Can you work these out from the model? Positions are in its coordinate system, mm. A direction names the side the tool comes from. Coordinates: 2 decimals unless noted, no trailing zeros. Order: outer loops, then holes, each group sorted by start corner. A loop starts at its lowest first (then second) coordinate and runs counter-clockwise, first axis right, second up. Notation, with made-up numbers: M 7.25,73 L 54.25,73 A8 ccw 54.25,87 Z; hole C 83,16 d10. An arc over 180 degrees is marked long. Answer as a JSON object with one key per item and string values.
from build123d import *

# Parameters (mm, degrees)
SKETCH1_R           = 5.0038
BOSS_EXTRUDE1_DEPTH = 12.0904
SKETCH1_5_R         = 6.604
SKETCH1_6_R         = 6.604
BOSS_EXTRUDE2_DEPTH = 3.302
SKETCH2_R           = 2.9972
CUT_EXTRUDE1_DEPTH  = 11.43
SKETCH3_R           = 5.2705
CUT_EXTRUDE2_DEPTH  = 2.9464
SKETCH4_W           = 1.623389838
SKETCH4_H           = 6.759688833
BOSS_EXTRUDE3_DEPTH = 12.192


with BuildPart() as part:
    # Sketch1 → Boss-Extrude1 (new body)
    with BuildSketch(Plane(origin=(0, 0, 0), x_dir=(1, 0, 0), z_dir=(0, 1, 0))):
        with Locations(Location((0, 0, 0), (0, 0, 270))):
            Circle(SKETCH1_R)
    extrude(amount=BOSS_EXTRUDE1_DEPTH)

    # Sketch1_5 → section 0 of loft1
    with BuildSketch(Plane(origin=(0, 0, 0), x_dir=(1, 0, 0), z_dir=(0, 1, 0)), mode=Mode.PRIVATE) as loft1_s0:
        Circle(SKETCH1_5_R)
    # loft up to a face of the part (loft1)
    loft([loft1_s0.sketch, Face(Wire([part.edges().sort_by_distance((3.647613218, 12.0904, -3.425336809))[0]]))])

    # Sketch1_6 → Boss-Extrude2 (add)
    with BuildSketch(Plane(origin=(0, 0, 0), x_dir=(1, 0, 0), z_dir=(0, 1, 0))):
        with Locations(Location((0, 0, 0), (0, 0, 270))):
            Circle(SKETCH1_6_R)
    extrude(amount=-BOSS_EXTRUDE2_DEPTH)

    # Sketch2 → Cut-Extrude1 (cut)
    with BuildSketch(Plane.XZ.offset(3.302)):
        with Locations(Location((0, 0, 0), (0, 0, 270))):
            Circle(SKETCH2_R)
    extrude(amount=-CUT_EXTRUDE1_DEPTH, mode=Mode.SUBTRACT)

    # Sketch3 → Cut-Extrude2 (cut)
    with BuildSketch(Plane.XZ.offset(3.302)):
        with Locations(Location((0, 0, 0), (0, 0, 270))):
            Circle(SKETCH3_R)
    extrude(amount=-CUT_EXTRUDE2_DEPTH, mode=Mode.SUBTRACT)

    # Sketch4 → Boss-Extrude3 (add)
    with BuildSketch(Plane.XZ.offset(0.3556)):
        with Locations((-2.310294919, 0.731856075)):
            Rectangle(SKETCH4_W, SKETCH4_H)
    extrude(amount=-BOSS_EXTRUDE3_DEPTH)


solid = part.part
Item 1: I want a section at B-B, the plane y = 4.25. Write out the boundary of the cut face in (x, z), plus the area to 3 significant figures.
Answers follow:
{"outline": "C 0,0 d12.08; hole M -1.5,-2.6 A3 ccw long -1.5,2.6 Z", "area": "92.0 mm^2"}
Item 2: Which directions (+Z, -Z, +X, -X, +Y, -Y) give clear straight access to the entire face, cutting with the end or side of a thin tool? Please do faces 4 (the flat face through (-5.4, -3.302, -0.5)), 5 (the cylindrical face through (2.996, 3.827, -0.088)).
Answers follow:
{"face 4": "+Z, -Z, +X, -X, -Y", "face 5": "-Y"}
Item 3: If we mould it in two halves opening along X, with no side actions, what happens to faces 1 (the flat face through (-2, -0.356, 0)), 2 (the flat face through (0, 12.09, 0)), 3 (the cylindrical face through (1.98, -1.63, 6.3))? For each: pulls with the +X half, pulls with the -X half, needs draft (parallel to the pull), parting line crosses it, or undercut.
Answers follow:
{"face 1": "undercut", "face 2": "needs draft", "face 3": "parting line crosses it"}
Item 4: I want a section at C-C, the plane y = 9.5. Write out the boundary of the cut face in (x, z).
Answers follow:
{"outline": "C 0,0 d10.69"}
Item 5: Please list where these lines run through material, in increasing order: line 1 (X direction, y = -2.5, z = 0); line 2 (X direction, y = -0.5, z = 1); line 3 (Y direction, x = -0.5, z = -4.25).
Answers follow:
{"line 1": "x = -6.6 to -5.27, 5.27 to 6.6", "line 2": "x = -6.53 to -5.17, 5.17 to 6.53", "line 3": "y = -0.36 to 12.09"}
Item 6: I want a section at A-A, the plane x = 0. Write out the boundary of the cut face in (y, z).
Answers follow:
{"outline": "M -3.3,-6.6 L 0,-6.6 L 12.09,-5 L 12.09,5 L 0,6.6 L -3.3,6.6 L -3.3,5.27 L -0.36,5.27 L -0.36,3 L 8.13,3 L 8.13,-3 L -0.36,-3 L -0.36,-5.27 L -3.3,-5.27 Z"}
Item 7: I'm going to push flat-ended pins straight in: pin 1 (1 mm diameter, centred on x = 4, y = 2, fed in from -Z); pin 2 (2 mm diameter, centred on y = 6.5, z = 4, fed in from +X); pin 3 (1.6 mm diameter, centred on y = 2, z = -1, fed in from +X). Where does each tip first touch, or does it pass through?
Answers follow:
{"pin 1": "stops at z = -5.29", "pin 2": "stops at x = 4.92", "pin 3": "stops at x = 6.4"}
Item 8: I want a section at D-D, the plane y = 1.5. Write out the boundary of the cut face in (x, z).
Answers follow:
{"outline": "C 0,0 d12.81; hole M -1.5,-2.6 A3 ccw long -1.5,2.6 Z"}
